Geometry check sheet. Reference: the model listing, model coordinates, mm. Face numbers are marked on the shaded views. A direction names the side the tool comes from. Coordinates: 2 decimals unless noted, no trailing zeros. Loops run counter-clockwise (first coordinate to the right, second up) from the corner with the lowest first, then second, coordinate; pieces in that order, holes last. Notation, with made-up numbers: M 42,43 L 98,43 A27 cw 98,74 Z; hole C 46.25,6.5 d1. An arc over 180 degrees is marked long. Use CSV: the item, a comma, the result in double quotes.
```python
from build123d import *

# Parameters (mm, degrees)
SKETCH1_W           = 130
SKETCH1_H           = 45
BOSS_EXTRUDE1_DEPTH = 50
SHELL1_T            = -2.5
SKETCH2_W           = 10
SKETCH2_H           = 40
BOSS_EXTRUDE2_DEPTH = 30
SKETCH5_W           = 2.5
SKETCH5_H           = 40
BOSS_EXTRUDE3_DEPTH = 47.5
SKETCH6_W           = 10
SKETCH6_H           = 40
BOSS_EXTRUDE4_DEPTH = 20
SKETCH7_W           = 10
SKETCH7_H           = 40
BOSS_EXTRUDE5_DEPTH = 25
SKETCH9_W           = 20
SKETCH9_H           = 10
CUT_EXTRUDE1_DEPTH  = 2.5
SKETCH11_W          = 15
SKETCH11_H          = 15
CUT_EXTRUDE2_DEPTH  = 12.5
SKETCH12_W          = 40
SKETCH12_H          = 5
CUT_EXTRUDE3_DEPTH  = 2.5
SKETCH20_R          = 1.5
CUT_EXTRUDE5_DEPTH  = 32.5
SKETCH21_R          = 1.5
CUT_EXTRUDE6_DEPTH  = 22.5
SKETCH22_R          = 1.5
CUT_EXTRUDE7_DEPTH  = 27.5
SKETCH24_R          = 3
CUT_EXTRUDE8_DEPTH  = 5
SKETCH25_W          = 40
SKETCH25_H          = 5
CUT_EXTRUDE9_DEPTH  = 2.5
SKETCH26_W          = 127.5
SKETCH26_H          = 2
CUT_EXTRUDE10_DEPTH = 1
SKETCH27_W          = 127.5
SKETCH27_H          = 2
CUT_EXTRUDE11_DEPTH = 1


with BuildPart() as part:
    # Sketch1 → Boss-Extrude1 (new body)
    with BuildSketch(Plane(origin=(0, 0, 0), x_dir=(1, 0, 0), z_dir=(0, 1, 0))):
        with Locations((6.071202057, 3.880136761)):
            Rectangle(SKETCH1_W, SKETCH1_H)
    extrude(amount=BOSS_EXTRUDE1_DEPTH)

    # Shell1
    shell1_openings = [part.faces().sort_by_distance(p)[0] for p in [
        (6.071202057, 50, -3.880136761),
    ]]
    offset(amount=SHELL1_T, openings=shell1_openings, kind=Kind.INTERSECTION)

    # Sketch2 → Boss-Extrude2 (add)
    with BuildSketch(Plane(origin=(0, 2.5, 0), x_dir=(1, 0, 0), z_dir=(0, 1, 0))):
        with Locations((63.571202057, 3.880136761)):
            Rectangle(SKETCH2_W, SKETCH2_H)
    extrude(amount=BOSS_EXTRUDE2_DEPTH)

    # Sketch5 → Boss-Extrude3 (add)
    with BuildSketch(Plane(origin=(0, 2.5, 0), x_dir=(1, 0, 0), z_dir=(0, 1, 0))):
        with Locations((29.821202057, 3.880136761)):
            Rectangle(SKETCH5_W, SKETCH5_H)
    extrude(amount=BOSS_EXTRUDE3_DEPTH)

    # Sketch6 → Boss-Extrude4 (add)
    with BuildSketch(Plane(origin=(0, 2.5, 0), x_dir=(1, 0, 0), z_dir=(0, 1, 0))):
        with Locations((23.571202057, 3.880136761)):
            Rectangle(SKETCH6_W, SKETCH6_H)
    extrude(amount=BOSS_EXTRUDE4_DEPTH)

    # Sketch7 → Boss-Extrude5 (add)
    with BuildSketch(Plane(origin=(0, 2.5, 0), x_dir=(1, 0, 0), z_dir=(0, 1, 0))):
        with Locations((-51.428797943, 3.880136761)):
            Rectangle(SKETCH7_W, SKETCH7_H)
    extrude(amount=BOSS_EXTRUDE5_DEPTH)

    # Sketch9 → Cut-Extrude1 (cut)
    with BuildSketch(Plane(origin=(-56.428797943, 0, 0), x_dir=(0, 0, -1), z_dir=(1, 0, 0))):
        with Locations((3.880136761, 32.5)):
            Rectangle(SKETCH9_W, SKETCH9_H)
    extrude(amount=-CUT_EXTRUDE1_DEPTH, mode=Mode.SUBTRACT)

    # Sketch11 → Cut-Extrude2 (cut)
    with BuildSketch(Plane.ZY.offset(-18.571202057)):
        with Locations((-3.880136761, 10)):
            Rectangle(SKETCH11_W, SKETCH11_H)
    extrude(amount=-CUT_EXTRUDE2_DEPTH, mode=Mode.SUBTRACT)

    # Sketch12 → Cut-Extrude3 (cut)
    with BuildSketch(Plane(origin=(-56.428797943, 0, 0), x_dir=(0, 0, -1), z_dir=(1, 0, 0))):
        with Locations((3.880136761, 47.5)):
            Rectangle(SKETCH12_W, SKETCH12_H)
    extrude(amount=-CUT_EXTRUDE3_DEPTH, mode=Mode.SUBTRACT)

    # Sketch20 → Cut-Extrude5 (cut)
    with BuildSketch(Plane(origin=(0, 32.5, 0), x_dir=(1, 0, 0), z_dir=(0, 1, 0))):
        with Locations(Location((63.571202057, -3.619863239, 0), (0, 0, 270))):
            Circle(SKETCH20_R)
        with Locations(Location((63.571202057, 11.380136761, 0), (0, 0, 270))):
            Circle(SKETCH20_R)
    extrude(amount=-CUT_EXTRUDE5_DEPTH, mode=Mode.SUBTRACT)

    # Sketch21 → Cut-Extrude6 (cut)
    with BuildSketch(Plane(origin=(0, 22.5, 0), x_dir=(1, 0, 0), z_dir=(0, 1, 0))):
        with Locations(Location((23.571202057, -8.619863239, 0), (0, 0, 270))):
            Circle(SKETCH21_R)
        with Locations(Location((23.571202057, 16.380136761, 0), (0, 0, 270))):
            Circle(SKETCH21_R)
    extrude(amount=-CUT_EXTRUDE6_DEPTH, mode=Mode.SUBTRACT)

    # Sketch22 → Cut-Extrude7 (cut)
    with BuildSketch(Plane(origin=(0, 27.5, 0), x_dir=(1, 0, 0), z_dir=(0, 1, 0))):
        with Locations(Location((-51.428797943, -8.619863239, 0), (0, 0, 270))):
            Circle(SKETCH22_R)
        with Locations(Location((-51.428797943, 16.380136761, 0), (0, 0, 270))):
            Circle(SKETCH22_R)
    extrude(amount=-CUT_EXTRUDE7_DEPTH, mode=Mode.SUBTRACT)

    # Sketch24 → Cut-Extrude8 (cut)
    with BuildSketch(Plane.XZ):
        with Locations(Location((-51.428797943, 8.619863239, 0), (0, 0, 270))):
            Circle(SKETCH24_R)
        with Locations(Location((-51.428797943, -16.380136761, 0), (0, 0, 270))):
            Circle(SKETCH24_R)
        with Locations(Location((23.571202057, 8.619863239, 0), (0, 0, 270))):
            Circle(SKETCH24_R)
        with Locations(Location((23.571202057, -16.380136761, 0), (0, 0, 270))):
            Circle(SKETCH24_R)
        with Locations(Location((63.571202057, 3.619863239, 0), (0, 0, 270))):
            Circle(SKETCH24_R)
        with Locations(Location((63.571202057, -11.380136761, 0), (0, 0, 270))):
            Circle(SKETCH24_R)
    extrude(amount=-CUT_EXTRUDE8_DEPTH, mode=Mode.SUBTRACT)

    # Sketch25 → Cut-Extrude9 (cut)
    with BuildSketch(Plane.ZY.offset(-28.571202057)):
        with Locations((-3.880136761, 47.5)):
            Rectangle(SKETCH25_W, SKETCH25_H)
    extrude(amount=-CUT_EXTRUDE9_DEPTH, mode=Mode.SUBTRACT)

    # Sketch26 → Cut-Extrude10 (cut)
    with BuildSketch(Plane(origin=(0, 0, 16.119863239), x_dir=(-1, 0, 0), z_dir=(0, 0, -1))):
        with Locations((-4.821202057, 46)):
            Rectangle(SKETCH26_W, SKETCH26_H)
    extrude(amount=-CUT_EXTRUDE10_DEPTH, mode=Mode.SUBTRACT)

    # Sketch27 → Cut-Extrude11 (cut)
    with BuildSketch(Plane.XY.offset(-23.880136761)):
        with Locations((4.821202057, 46)):
            Rectangle(SKETCH27_W, SKETCH27_H)
    extrude(amount=-CUT_EXTRUDE11_DEPTH, mode=Mode.SUBTRACT)


solid = part.part
```
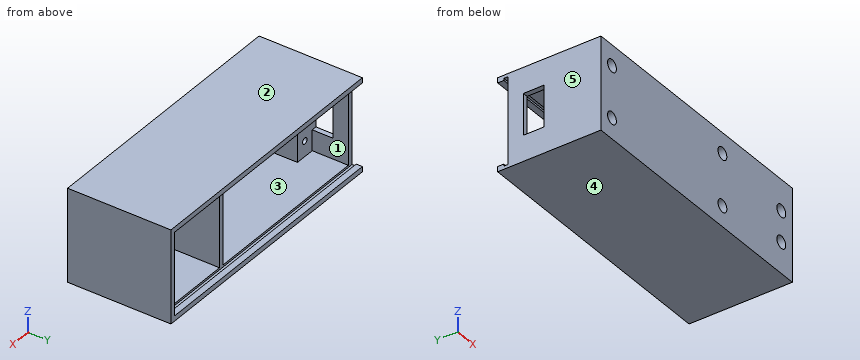
1. Set-up check for the marked faces 1 and 2: record each of +Z, -Z, +X, -X, +Y, -Y from which the full face is reachable in a straight line by a thin tool's end or side.
The answers:
face 1,"+Y"
face 2,"+Z, +X, -X, +Y, -Y"
2. Release check for a two-part mould opening along Z. For the marked faces 3, 4 and 5 record: +Z half, -Z half, draft (parallel to the pull), parting line (faces both ways), or undercut.
The answers:
face 3,"undercut"
face 4,"-Z half"
face 5,"draft"
3. Gauge pin test, flat ends, axial feed: P1, Ø8, axis at x = 22, z = 2, coming from the +Y side; P2, Ø10, axis at x = -50.5, z = -10, coming from the +Y side; P3, Ø5, axis at x = -51, z = 8.5, coming from the -Y side. Record the tip position at first contact, or that the pin passes through.
The answers:
P1,"y = 22.5"
P2,"y = 27.5"
P3,"y = 5"
4. Section check D-D, the plane y = 24.5. Record the cut outline in (x, z), plus the area to 3 significant figures.
The answers:
outline,"M -58.93,-26.38 L 71.07,-26.38 L 71.07,18.62 L -58.93,18.62 Z; hole C -51.43,-16.38 d3; hole C -51.43,8.62 d3; hole M -46.43,-23.88 L 28.57,-23.88 L 28.57,16.12 L -46.43,16.12 Z; hole M 31.07,-23.88 L 58.57,-23.88 L 58.57,16.12 L 31.07,16.12 Z; hole C 63.57,-11.38 d3; hole C 63.57,3.62 d3"
area,"1,720 mm^2"
5. Section check C-C, the plane z = 13.5. Record the cut outline in (x, y).
The answers:
outline,"M -58.93,0 L 71.07,0 L 71.07,50 L 68.57,50 L 68.57,32.5 L 58.57,32.5 L 58.57,2.5 L 31.07,2.5 L 31.07,45 L 28.57,45 L 28.57,22.5 L 18.57,22.5 L 18.57,2.5 L -46.43,2.5 L -46.43,27.5 L -56.43,27.5 L -56.43,45 L -58.93,45 Z"
6. Section check A-A, the plane z = -3. Record the cut outline in (x, y), plus the area to 3 significant figures.
The answers:
outline,"M -58.93,0 L 71.07,0 L 71.07,50 L 68.57,50 L 68.57,32.5 L 58.57,32.5 L 58.57,2.5 L -46.43,2.5 L -46.43,27.5 L -58.93,27.5 Z; M -58.93,37.5 L -56.43,37.5 L -56.43,45 L -58.93,45 Z; M 18.57,17.5 L 31.07,17.5 L 31.07,45 L 28.57,45 L 28.57,22.5 L 18.57,22.5 Z"
area,"1,190 mm^2"
7. Thickness scan on line 1 (X direction, y = 40, z = -19); line 2 (X direction, y = 10.5, z = -13.5); line 3 (Z direction, x = -21.5, y = 18.5). Record the ranges inside material, lowest first. Write a range as [from, to].
The answers:
line 1,"[-58.93, -56.43], [28.57, 31.07], [68.57, 71.07]"
line 2,"[-58.93, -46.43], [18.57, 31.07], [58.57, 71.07]"
line 3,"[-26.38, -23.88], [16.12, 18.62]"
8. Section check B-B, the plane y = 34. Record the cut outline in (x, z), plus the area to 3 significant figures.
The answers:
outline,"M -58.93,-26.38 L 71.07,-26.38 L 71.07,18.62 L -58.93,18.62 L -58.93,6.12 L -56.43,6.12 L -56.43,16.12 L 28.57,16.12 L 28.57,-23.88 L -56.43,-23.88 L -56.43,-13.88 L -58.93,-13.88 Z; hole M 31.07,-23.88 L 68.57,-23.88 L 68.57,16.12 L 31.07,16.12 Z"
area,"900 mm^2"
